from build123d import *

# Parameters (mm, degrees)
F0_R     = 75
F0_W     = 100
F0_H     = 5
F1_DEPTH = 5
F2_DEPTH = 50
F4_DEPTH = 3


with BuildPart() as f1:
    # F0 (on Top) → F1 (new body)
    with BuildSketch(Plane.XY):
        with BuildLine():
            ThreePointArc((-50, 62.449979984), (-34.6410161514, -72.1110255093), (80, 0))
            ThreePointArc((80, 0), (72.1110255093, 34.6410161514), (50, 62.449979984))
            ThreePointArc((50, 62.449979984), (0, 80), (-50, 62.449979984))
        make_face()
        Circle(F0_R, mode=Mode.SUBTRACT)
        with BuildLine():
            ThreePointArc((-50, 62.449979984), (0, 80), (50, 62.449979984))
            Line((50, 62.449979984), (50, 85))
            Line((50, 85), (-50, 85))
            Line((-50, 85), (-50, 62.449979984))
        make_face()
        with Locations((0, 87.5)):
            Rectangle(F0_W, F0_H)
    extrude(amount=F1_DEPTH)

    # F0 (on Top) → F2 (join)
    with BuildSketch(Plane.XY):
        with Locations((0, 87.5)):
            Rectangle(F0_W, F0_H)
    extrude(amount=F2_DEPTH)

    # F3 (on face) → F4 (join)
    with BuildSketch(Plane.YZ.offset(50)):
        Polygon((85, 5), (85, 50), (62.449979984, 5), align=None)
    extrude(amount=-F4_DEPTH)

    # F5: F1 across plane


with BuildPart() as f1_1:
    add(f1.part)
    add(f1.part.mirror(Plane.YZ))


solid = f1_1.part
Could you check a few things on this model? Use its own coordinates, in mm. A direction names the side the tool comes from. Round coordinates to 2 decimals unless told otherwise and drop trailing zeros. Write each loop counter-clockwise with the first axis right and the second up, starting at its lowest first coordinate (ties: lowest second). Pieces come first, ordered by that corner, then holes. Notation, with made-up numbers: (-18, -15) -> (23, -15) arc R24 ccw to (23, 15) -> close; hole circle Ø5 at (-14, 4). An arc over 180 degrees is marked (long way). Use a Markdown table: item, result.
1. If we section it at B-B (y = -20.5): List the corners of the cut face in (x, z) for me, then the cut area to 3 significant figures.
Answer key:
| item | result |
|---|---|
| outline | (-77.33, 0) -> (-72.14, 0) -> (-72.14, 5) -> (-77.33, 5) -> close; (72.14, 0) -> (77.33, 0) -> (77.33, 5) -> (72.14, 5) -> close |
| area | 51.8 mm^2 |
2. Please list where these lines run through material, in increasing order: probe 1 along X at (y, z) = (0, 2); probe 2 along Y at (x, z) = (0, 2.9); probe 3 along X at (y, z) = (64, 6).
Answer key:
| item | result |
|---|---|
| probe 1 | x = -80 to -75, 75 to 80 |
| probe 2 | y = -80 to -75, 75 to 90 |
| probe 3 | x = -50 to -47, 47 to 50 |
3. If we section it at C-C (z = 20): List the corners of the cut face in (x, y) for me.
Answer key:
| item | result |
|---|---|
| outline | (-50, 69.97) -> (-47, 69.97) -> (-47, 85) -> (47, 85) -> (47, 69.97) -> (50, 69.97) -> (50, 90) -> (-50, 90) -> close |
4. If we section it at D-D (y = 33): List the corners of the cut face in (x, z) for me.
Answer key:
| item | result |
|---|---|
| outline | (-72.88, 0) -> (-67.35, 0) -> (-67.35, 5) -> (-72.88, 5) -> close; (67.35, 0) -> (72.88, 0) -> (72.88, 5) -> (67.35, 5) -> close |
5. If we section it at A-A (x = 0): List the corners of the cut face in (y, z) for me.
Answer key:
| item | result |
|---|---|
| outline | (-80, 0) -> (-75, 0) -> (-75, 5) -> (-80, 5) -> close; (75, 0) -> (90, 0) -> (90, 50) -> (85, 50) -> (85, 5) -> (75, 5) -> close |
6. We'd pull the mould along Y, two halves only. Please class faces 6 (the face through (-9.764, 74.362, 2.465)), 7 (the face through (-1, 90, 25)), 8 (the face through (47, 79, 18)): +Y half, -Y half, draft (parallel to the pull), parting line (faces both ways), or undercut.
Answer key:
| item | result |
|---|---|
| face 6 | undercut |
| face 7 | +Y half |
| face 8 | draft |
7. Which directions (+Z, -Z, +X, -X, +Y, -Y) give clear straight access to the entire face, cutting with the end or side of a thin tool? Please do faces 1 (the face through (-1, 85, 27)), 2 (the face through (-12, 75, 0)), 3 (the face through (-50, 79, 20)), 4 (the face through (-2.762, -79.952, 2.465)), 5 (the face through (50, 79, 20)).
Answer key:
| item | result |
|---|---|
| face 1 | +Z, -Y |
| face 2 | -Z, +X, -X, +Y, -Y |
| face 3 | +Z, -Z, -X, +Y |
| face 4 | +Z, -Z |
| face 5 | +Z, -Z, +X, +Y |
8. For pin 1 Ø11.5 at (y, z) = (77, 29) entering from +X; pin 2 Ø8.5 at (y, z) = (81, 23) entering from -X; pin 3 Ø4 at (x, z) = (1, 10) entering from -Y, each with a flat end and sliding along its axis, tell me the tip position at first contact or that it passes through.
Answer key:
| item | result |
|---|---|
| pin 1 | stops at x = 50 |
| pin 2 | stops at x = -50 |
| pin 3 | stops at y = 85 |
